Geometry check sheet. Reference: the model listing, model coordinates, mm. Round coordinates to 2 decimals unless told otherwise and drop trailing zeros. Order: outer loops, then holes, each group sorted by start corner. A loop starts at its lowest first (then second) coordinate and runs counter-clockwise, first axis right, second up. Notation, with made-up numbers: (-9, 75) -> (32, 75) arc R34 cw to (32, 106) -> close; hole circle Ø5 at (17, 31.5). An arc over 180 degrees is marked (long way). Use a Markdown table: item, result. Add a question column.
Item 1: Sectioned sample at C-C, the plane y = 452.5. Record the cut outline in (x, z).
Item 2: Material ranges on probe 1 along Z at (x, y) = (0, 549); probe 2 along X at (y, z) = (689, 2); probe 3 along X at (y, z) = (226, 1), recorded low to high. Write a range as [from, to].
Item 3: Sectioned sample at A-A, the plane z = 0. Record the cut outline in (x, y).
Item 4: Sectioned sample at B-B, the plane x = -10.5. Record the cut outline in (y, z).
Item 5: Gauge pin test, flat ends, axial feed: pin 1 Ø2 at (y, z) = (205.5, -13.5) entering from +X; pin 2 Ø12 at (y, z) = (514, 12.5) entering from -X; pin 3 Ø3 at (y, z) = (397, -9) entering from -X. Record the tip position at first contact, or that the pin passes through.
Item 6: Mould release check, pull along Z, two halves, no side actions. Record for faces 1 (the cylindrical face through (-2.343, 386.334, -17.847)), 2 (the flat face through (-7, 0, -17)), 3 (the cylindrical face through (15.12, 375.67, 11.59)): pulls with the +Z half, pulls with the -Z half, needs draft (parallel to the pull), parting line crosses it, or undercut.
Autodesk Inventor part; units mm, degrees
ref_plane "Work Plane1" through (0, 0, 29.95) normal (0, 0, 1) x (1, 0, 0)
ref_plane "YZ Plane" through (0, 0, 0) normal (1, 0, 0) x (0, 1, 0)
ref_plane "XZ Plane" through (0, 0, 0) normal (0, 1, 0) x (-1, 0, 0)
sketch "Sketch1" plane through (0, 0, 0) normal (0, 1, 0) x (-1, 0, 0)
  circle A0 centre (0, 0) radius 19.05
  dimension "d0" = 38.1
extrude "Extrusion1" add sketch "Sketch1" along normal blind 762
sketch "Sketch2" plane through (0, 762, 0) normal (0, 1, 0) x (1, 0, 0)
  circle A0 centre (0, 0) radius 18
  dimension "d3" = 36
extrude "Extrusion2" cut sketch "Sketch2" along normal through all both and the other way through all
ref_plane "Work Plane1" through (0, 0, 29.95) normal (0, 0, 1) x (1, 0, 0)
sketch "Sketch3" plane through (0, 0, 29.95) normal (0, 0, 1) x (1, 0, 0)
  line L0 (0, 0) -> (0, 100)
  line L1 (-18, 100) -> (18, 100)
  line L2 (-2.3812, 100) -> (2.3812, 100)
  line L3 (2.3812, 100) -> (2.3813, 150)
  line L4 (2.3813, 150) -> (-2.3812, 150)
  line L5 (-2.3812, 150) -> (-2.3812, 100)
  dimension "d15" = 4.7625
  dimension "d16" = 50
extrude "Extrusion3" cut sketch "Sketch3" against normal blind 29.95
sketch "Sketch4" plane through (0, 0, 0) normal (0, -1, 0) x (1, 0, 0)
  circle A0 centre (0, 0) radius 19
  circle A1 centre (0, 0) radius 29.95
  dimension "d11" = 38
properties part number "Shaft connecting chassis updated 1-19"
Found:
| question | item | result |
|---|---|---|
| 1 | outline | circle Ø38.1 at (0, 0); hole circle Ø36 at (0, 0) |
| 2 | probe 1 | z = [-19.05, -18], [18, 19.05] |
| 2 | probe 2 | x = [-18.94, -17.89], [17.89, 18.94] |
| 2 | probe 3 | x = [-19.02, -17.97], [17.97, 19.02] |
| 3 | outline | (-19.05, 0) -> (-18, 0) -> (-18, 762) -> (-19.05, 762) -> close; (18, 0) -> (19.05, 0) -> (19.05, 762) -> (18, 762) -> close |
| 4 | outline | (0, -15.9) -> (762, -15.9) -> (762, -14.62) -> (0, -14.62) -> close; (0, 14.62) -> (762, 14.62) -> (762, 15.9) -> (0, 15.9) -> close |
| 5 | pin 1 | stops at x = 14.38 |
| 5 | pin 2 | stops at x = -17.91 |
| 5 | pin 3 | stops at x = -17.51 |
| 6 | face 1 | undercut |
| 6 | face 2 | needs draft |
| 6 | face 3 | parting line crosses it |
